from build123d import *

# Parameters (mm, degrees)
SKETCH2_W           = 132
SKETCH2_H           = 19
BOSS_EXTRUDE1_DEPTH = 20
SKETCH3_R           = 7.5
BOSS_EXTRUDE2_DEPTH = 3
SKETCH4_W           = 1
SKETCH4_H           = 4
BOSS_EXTRUDE3_DEPTH = 2
CUT_EXTRUDE1_REACH  = 181
SKETCH5_R           = 1.45
FILLET1_R           = 2
SKETCH6_R           = 2
CUT_EXTRUDE2_DEPTH  = 10


with BuildPart() as part:
    # Sketch2 → Boss-Extrude1 (new body)
    with BuildSketch(Plane(origin=(0, 0, 0), x_dir=(0, 0, -1), z_dir=(1, 0, 0))):
        with BuildLine():
            Line((88, 2.5), (88, -2.5))
            ThreePointArc((88, -2.5), (85.071067812, -9.571067812), (78, -12.5))
            Line((78, -12.5), (-88, -12.5))
            Line((-88, -12.5), (-88, -9.5))
            Line((-88, -9.5), (-88, 9.5))
            Line((-88, 9.5), (-88, 12.5))
            Line((-88, 12.5), (78, 12.5))
            ThreePointArc((78, 12.5), (85.071067812, 9.571067812), (88, 2.5))
        make_face()
        with BuildLine():
            ThreePointArc((61.514718626, -3), (79, 0), (61.514718626, 3))
            Line((61.514718626, 3), (58.2, 3))
            Line((58.2, 3), (58.2, -3))
            Line((58.2, -3), (61.514718626, -3))
        make_face(mode=Mode.SUBTRACT)
        with Locations((-19, 0)):
            Rectangle(SKETCH2_W, SKETCH2_H, mode=Mode.SUBTRACT)
        Polygon((-85, 7.984540751), (36.47154627, -9.5), (47, -9.5), (47, -7.984540751), (-74.47154627, 9.5), (-85, 9.5), align=None)
    extrude(amount=BOSS_EXTRUDE1_DEPTH)

    # Sketch3 → Boss-Extrude2 (add)
    with BuildSketch(Plane.XY.offset(88)):
        with Locations((10, 0)):
            Circle(SKETCH3_R)
    extrude(amount=BOSS_EXTRUDE2_DEPTH)

    # Sketch4 → Boss-Extrude3 (add)
    with BuildSketch(Plane.XY.offset(91)):
        with Locations((5, 0)):
            Rectangle(SKETCH4_W, SKETCH4_H)
        with Locations((15, 0)):
            Rectangle(SKETCH4_W, SKETCH4_H)
    extrude(amount=BOSS_EXTRUDE3_DEPTH)

    # Sketch5 → Cut-Extrude1 (cut, up to next)
    with BuildSketch(Plane.XY.offset(91), mode=Mode.PRIVATE) as cut_extrude1_sk1:
        with Locations((10, 0)):
            Circle(SKETCH5_R)
    cut_extrude1_tool1 = extrude(cut_extrude1_sk1.sketch, amount=-CUT_EXTRUDE1_REACH, mode=Mode.PRIVATE) & part.part
    add(cut_extrude1_tool1.solids().sort_by_distance((10, 0, 91))[0], mode=Mode.SUBTRACT)

    # Fillet1
    fillet1_edges = [part.edges().sort_by_distance(p)[0] for p in [
        (10, 9.5, -47),
        (10, -9.5, 85),
    ]]
    fillet(fillet1_edges, radius=FILLET1_R)

    # Sketch6 → Cut-Extrude2 (cut)
    with BuildSketch(Plane(origin=(0, -9.5, 0), x_dir=(1, 0, 0), z_dir=(0, 1, 0))):
        with Locations((10, -53)):
            Circle(SKETCH6_R)
        with Locations((10, -68)):
            Circle(SKETCH6_R)
        with Locations((10, -38)):
            Circle(SKETCH6_R)
    extrude(amount=-CUT_EXTRUDE2_DEPTH, mode=Mode.SUBTRACT)


solid = part.part
Work out the finished part from the listing and answer in its coordinate system (mm). A direction names the side the tool comes from. Give positions to 0.01 mm unless a question says otherwise; leave off trailing zeros. Loops run counter-clockwise (first coordinate to the right, second up) from the corner with the lowest first, then second, coordinate; pieces in that order, holes last. Notation, with made-up numbers: (24, 51.25) - (79, 51.25) arc R27 ccw to (79, 72.25) - close; hole circle Ø1 at (46.5, -0.5). An arc over 180 degrees is marked (long way). Answer in a Markdown table with one row per item.
(1) Section C-C (z = 78) is taken. Give the vertices of the cut face in (x, y), and give its area (3 significant figures).
Results list:
| item | result |
|---|---|
| outline | (0, -12.5) - (20, -12.5) - (20, -9.5) - (0, -9.5) - close; (0, 6.98) - (20, 6.98) - (20, 12.5) - (0, 12.5) - close |
| area | 170 mm² |
(2) Consider L1, parallel to Y at x = 2.5, z = -70; L2, parallel to Y at x = 5.5, z = 24.5; L3, parallel to Y at x = 11.5, z = -5.5. Determine where each line is inside the solid, lowest interval first. Write a range as [from, to].
Results list:
| item | result |
|---|---|
| L1 | y = [-12.5, -9], [9, 12.5] |
| L2 | y = [-12.5, -9.5], [-0.72, 2.31], [9.5, 12.5] |
| L3 | y = [-12.5, -9.5], [-5.04, -2.01], [9.5, 12.5] |
(3) Flat-ended cylindrical pins translate along their axes: pin 1 Ø1.1 at (x, z) = (5, 92.5) entering from +Y; pin 2 Ø12 at (x, y) = (9.5, -1.5) entering from +Z; pin 3 Ø1 at (x, y) = (16, 5) entering from +Z; pin 4 Ø1 at (y, z) = (-0.5, 92) entering from -X. Find the tip coordinate at first contact, or state that the pin passes through.
Results list:
| item | result |
|---|---|
| pin 1 | stops at y = 2 |
| pin 2 | stops at z = 93 |
| pin 3 | stops at z = 91 |
| pin 4 | stops at x = 4.5 |
(4) For a pull along Z with two mould halves and no side action, classify faces 1 (the face through (10, -12.5, 4)), 2 (the face through (10, 9.5, 16)), 3 (the face through (9.86, 0.635, 12.885)), 4 (the face through (10, -9, 88)) as pulls with the +Z half, pulls with the -Z half, needs draft (parallel to the pull), parting line crosses it, or undercut.
Results list:
| item | result |
|---|---|
| face 1 | needs draft |
| face 2 | undercut |
| face 3 | undercut |
| face 4 | pulls with the +Z half |
(5) Section A-A (z = -70) is taken. Give the vertices of the cut face in (x, y), and give its area (3 significant figures).
Results list:
| item | result |
|---|---|
| outline | (0, -12.5) - (20, -12.5) - (20, -9) - (0, -9) - close; (0, 9) - (20, 9) - (20, 12.5) - (0, 12.5) - close |
| area | 140 mm² |
(6) A tool of negligible diameter and unlimited length cuts with its end or side. For faces 5 (the face through (10, 2, 85)), 6 (the face through (9.86, 9.65, -84.99)), 7 (the face through (8.55, 0.06, 88.04)), 8 (the face through (10, 12.5, 6)), 9 (the face through (10, -11, 66)), from which of +Z, -Z, +X, -X, +Y, -Y can it reach the whole face along a straight path? Write none if from no direction.
Results list:
| item | result |
|---|---|
| face 5 | +X, -X |
| face 6 | -Z, +X, -X, +Y |
| face 7 | +Z |
| face 8 | +Z, -Z, +X, -X, +Y |
| face 9 | -Y |
(7) Section B-B (z = 38) is taken. Give the vertices of the cut face in (x, y), and give its area (3 significant figures).
Results list:
| item | result |
|---|---|
| outline | (0, -12.5) - (8, -12.5) - (8, -9.5) - (0, -9.5) - close; (0, 1.22) - (20, 1.22) - (20, 4.25) - (0, 4.25) - close; (0, 9.5) - (20, 9.5) - (20, 12.5) - (0, 12.5) - close; (12, -12.5) - (20, -12.5) - (20, -9.5) - (12, -9.5) - close |
| area | 169 mm² |
